```python
from build123d import *

# Parameters (mm, degrees)
SKETCH1_R              = 3.45
SKETCH1_R_2            = 2.5
BOSS_EXTRUDE1_DEPTH    = 2.2
BOSS_EXTRUDE4_START    = 1.7
SKETCH1_9_R            = 3.45
SKETCH1_9_R_2          = 2.5
BOSS_EXTRUDE4_DEPTH    = 1.7
BOSS_EXTRUDE5_START    = 1.7
BOSS_EXTRUDE5_DEPTH    = 1.7
MIRROR3_START          = 1.7
MIRROR3_COPY_1_DEPTH   = 1.7
FILLET1_R              = 1
SKETCH2_R              = 2.5
F_0ZVARIANCEBOSS_DEPTH = 0.2


with BuildPart() as part:
    # Sketch1 → Boss-Extrude1 (new body)
    with BuildSketch(Plane.XY):
        with Locations((-5.15, 0)):
            Circle(SKETCH1_R)
        with Locations((-5.15, 0)):
            Circle(SKETCH1_R_2, mode=Mode.SUBTRACT)
    extrude(amount=-BOSS_EXTRUDE1_DEPTH)

    # Sketch1<9> → Boss-Extrude4 (add)
    # profile 1 of 2: a face of its own
    with BuildSketch(Plane.XY.offset(BOSS_EXTRUDE4_START)):
        with Locations((-5.15, 0)):
            Circle(SKETCH1_9_R)
        with Locations((-5.15, 0)):
            Circle(SKETCH1_9_R_2, mode=Mode.SUBTRACT)
    # profile 2 of 2: a face of its own
    with BuildSketch(Plane.XY.offset(BOSS_EXTRUDE4_START)):
        with Locations((-5.15, 0)):
            Circle(SKETCH1_9_R_2)
    extrude(amount=-BOSS_EXTRUDE4_DEPTH)

    # Sketch1<10> → Boss-Extrude5 (add)
    with BuildSketch(Plane.XY.offset(BOSS_EXTRUDE5_START)):
        with BuildLine():
            Line((-7.589518395, 2.439518395), (-8.6, 3.45))
            Line((-8.6, 3.45), (-9.307106781, 4.157106781))
            Line((-9.307106781, 4.157106781), (-16.963017409, 2.178419472))
            ThreePointArc((-16.963017409, 2.178419472), (-18.65, 0), (-16.963017409, -2.178419472))
            Line((-16.963017409, -2.178419472), (-9.307106781, -4.157106781))
            Line((-9.307106781, -4.157106781), (-8.6, -3.45))
            Line((-8.6, -3.45), (-7.589518395, -2.439518395))
            ThreePointArc((-7.589518395, -2.439518395), (-8.6, 0), (-7.589518395, 2.439518395))
        make_face()
    boss_extrude5 = extrude(amount=-BOSS_EXTRUDE5_DEPTH)

    # Mirror2: Boss-Extrude5 across plane
    add(boss_extrude5.mirror(Plane(origin=(-2.575, 2.575, 0), x_dir=(0, 0, 1), z_dir=(0.7071067811865476, -0.7071067811865475, 0))))

    # Mirror3: Boss-Extrude5 across plane
    add(boss_extrude5.mirror(Plane(origin=(-2.575, -2.575, 0), x_dir=(0, 0, 1), z_dir=(0.7071067811865476, 0.7071067811865475, 0))))

    # Mirror3 copy 1 sketch → Mirror3 copy 1 (add)
    with BuildSketch(Plane(origin=(-10.3, 0, 0), x_dir=(-1, 0, 0), z_dir=(0, 0, 1)).offset(MIRROR3_START)):
        with BuildLine():
            Line((-7.589518395, 2.439518395), (-8.6, 3.45))
            Line((-8.6, 3.45), (-9.307106781, 4.157106781))
            Line((-9.307106781, 4.157106781), (-16.963017409, 2.178419472))
            ThreePointArc((-16.963017409, 2.178419472), (-18.65, 0), (-16.963017409, -2.178419472))
            Line((-16.963017409, -2.178419472), (-9.307106781, -4.157106781))
            Line((-9.307106781, -4.157106781), (-8.6, -3.45))
            Line((-8.6, -3.45), (-7.589518395, -2.439518395))
            ThreePointArc((-7.589518395, -2.439518395), (-8.6, 0), (-7.589518395, 2.439518395))
        make_face()
    extrude(amount=-MIRROR3_COPY_1_DEPTH)

    # Fillet1
    fillet1_edges = [part.edges().sort_by_distance(p)[0] for p in [
        (-9.307106781, 4.157106781, 0.85),
        (-9.307106781, -4.157106781, 0.85),
        (-0.992893219, -4.157106781, 0.85),
        (-0.992893219, 4.157106781, 0.85),
    ]]
    fillet(fillet1_edges, radius=FILLET1_R)

    # Sketch2 → 0ZvarianceBoss (add)
    with BuildSketch(Plane(origin=(0, 0, 0), x_dir=(-1, 0, 0), z_dir=(0, 0, -1))):
        with Locations(Location((5.15, 0, 0), (0, 0, 180))):
            Circle(SKETCH2_R)
    extrude(amount=F_0ZVARIANCEBOSS_DEPTH)


solid = part.part
```
The listing builds one solid part. Answer for the finished solid, in the listing's coordinates (mm). A direction names the side the tool comes from. Give positions to 0.01 mm unless a question says otherwise; leave off trailing zeros. Write each loop counter-clockwise with the first axis right and the second up, starting at its lowest first coordinate (ties: lowest second). Pieces come first, ordered by that corner, then holes. Notation, with made-up numbers: M 18.5,41 L 24.5,41 A30 cw 24.5,68 Z; hole C 34,8.25 d6. An arc over 180 degrees is marked long. Write each question's results on one line, items separated by ' | '.
Q1. A flat-ended cylindrical pin translates along its axis: P1, Ø2, axis at x = -3.5, y = 5, coming from the -Z side. Find the tip coordinate at first contact, or state that the pin passes through.
Output values:
P1: z = 0
Q2. A tool of negligible diameter and unlimited length cuts with its end or side. For faces 1 (the flat face through (-3, 3, 0)), 2 (the cylindrical face through (-18.65, 0.04, 0.86)), from which of +Z, -Z, +X, -X, +Y, -Y can it reach the whole face along a straight path? Write none if from no direction.
Output values:
face 1: -Z | face 2: +Z, -Z, -X
Q3. Consider L1, parallel to Y at x = -5.15, z = -1.8; L2, parallel to X at y = 0, z = -0.6; L3, parallel to Z at x = -8.5, y = 1. Determine where each line is inside the solid, lowest interval first. Write a range as from..to.
Output values:
L1: -3.45..-2.5, 2.5..3.45 | L2: -8.6..-7.65, -2.65..-1.7 | L3: 0..1.7
Q4. Section B-B, the plane z = 0.6 is taken. Write down the section's boundary in (x, y).
Output values:
outline: M -16.96,-2.18 L -9.88,-4.01 A1 cw -9.16,-4.73 L -7.33,-11.81 A2.25 ccw -2.97,-11.81 L -1.14,-4.73 A1 cw -0.42,-4.01 L 6.66,-2.18 A2.25 ccw 6.66,2.18 L -0.42,4.01 A1 cw -1.14,4.73 L -2.97,11.81 A2.25 ccw -7.33,11.81 L -9.16,4.73 A1 cw -9.88,4.01 L -16.96,2.18 A2.25 ccw Z
Q5. Section C-C, the plane x = -5.15 is taken. Write down the section's boundary in (y, z).
Output values:
outline: M -13.5,0 L -3.45,0 L -3.45,-2.2 L -2.5,-2.2 L -2.5,-0.2 L 2.5,-0.2 L 2.5,-2.2 L 3.45,-2.2 L 3.45,0 L 13.5,0 L 13.5,1.7 L -13.5,1.7 Z
Q6. Section A-A, the plane y = 0 is taken. Write down the section's boundary in (x, z).
Output values:
outline: M -18.65,0 L -8.6,0 L -8.6,-2.2 L -7.65,-2.2 L -7.65,-0.2 L -2.65,-0.2 L -2.65,-2.2 L -1.7,-2.2 L -1.7,0 L 8.35,0 L 8.35,1.7 L -18.65,1.7 Z
Q7. Section D-D, the plane y = 8 is taken. Write down the section's boundary in (x, z), then the cut area to 3 significant figures.
Output values:
outline: M -8.31,0 L -1.99,0 L -1.99,1.7 L -8.31,1.7 Z | area: 10.8 mm2
